Autodesk Inventor part; units mm, degrees
ref_plane "YZ Plane" through (0, 0, 0) normal (1, 0, 0) x (0, 1, 0)
ref_plane "XZ Plane" through (0, 0, 0) normal (0, 1, 0) x (-1, 0, 0)
ref_plane "XY Plane" through (0, 0, 0) normal (0, 0, 1) x (1, 0, 0)
sketch "Sketch1" plane through (0, 0, 0) normal (0, 0, 1) x (1, 0, 0)
  line L0 (-7.3323, 0) -> (-3.6662, 6.35)
  line L1 (-3.6662, 6.35) -> (3.6662, 6.35)
  line L2 (3.6662, 6.35) -> (7.3323, 0)
  line L3 (7.3323, 0) -> (3.6662, -6.35)
  line L4 (3.6662, -6.35) -> (-3.6662, -6.35)
  line L5 (-3.6662, -6.35) -> (-7.3323, 0)
  circle A0 centre (0, 6.35) radius 1.524
  circle A1 centre (-5.4993, 3.175) radius 1.524
  circle A2 centre (-5.4993, -3.175) radius 1.524
  circle A3 centre (0, -6.35) radius 1.524
  circle A4 centre (5.4993, -3.175) radius 1.524
  circle A5 centre (5.4993, 3.175) radius 1.524
  circle A6 centre (0, 0) radius 2.9337
  point P0 (6.2613, 1.8552)
  point P1 (4.7373, 4.4948)
  point P2 (1.524, 6.35)
  point P3 (-1.524, 6.35)
  point P4 (-4.7373, 4.4948)
  point P5 (-6.2613, 1.8552)
  point P6 (-6.2613, -1.8552)
  point P7 (-4.7373, -4.4948)
  point P8 (-1.524, -6.35)
  point P9 (1.524, -6.35)
  point P10 (4.7373, -4.4948)
  point P11 (6.2613, -1.8552)
  dimension "d0" = 12.7
  dimension "d1" = 3.048
  dimension "d4" = 360
  dimension "d6" = 5.8674
extrude "Extrusion1" add sketch "Sketch1" along normal mid plane 60.325 contours L0 A1 L1 A0 L2 A5 L3 A4 L4 A3 L5 A2
properties part number "Configurable Kitbot Churro" material "Aluminum"
For this review, take the finished solid that the model builds, in its own axes (mm). Give positions to 0.01 mm unless a question says otherwise; leave off trailing zeros. Loops run counter-clockwise (first coordinate to the right, second up) from the corner with the lowest first, then second, coordinate; pieces in that order, holes last. Notation, with made-up numbers: M 78,-2.5 L 109,-2.5 A28 ccw 109,30.5 Z; hole C 17,-30.75 d4. An arc over 180 degrees is marked long. Put each result on its own line as item: value. Start each with the question number.
(1) Add section D-D, the plane y = 3.5. Write out the cut boundary in (x, z), then the cut area to 3 significant figures.
(2) Add section A-A, the plane z = 11. Write out the cut boundary in (x, y) (3 decimals).
(3) Wall thickness on L1, parallel to Y at x = 0, z = -17; L2, parallel to Y at x = -2.5, z = -21; L3, parallel to X at y = 5.75, z = 21.5: over which ranges is each line inside the solid? List them lowest first.
(4) For pin 1 (2 mm diameter, centred on y = -4.5, z = 4.5, fed in from -X); pin 2 (1.5 mm diameter, centred on y = 3.5, z = 22, fed in from +X), all flat-tipped, find the tip position at first contact; note any pin that passes through.
(5) Add section B-B, the plane x = 0. Write out the cut boundary in (y, z), then the cut area to 3 significant figures.
(6) Add section C-C, the plane x = -2.25. Write out the cut boundary in (y, z), then the cut area to 3 significant figures.
(7) The part is to be moulded in two halves that separate along Y. For faces 1 (the flat face through (3.2, 0.1, -30.162)), 2 (the flat face through (4.21, -5.41, -0.42)), 3 (the cylindrical face through (4.2, 2.38, -0.42)), 4 (the cylindrical face through (-4.163, 2.442, -0.422)), say which applies: +Y half, -Y half, draft (parallel to the pull), parting line (faces both ways), or undercut.
Result:
1. outline: M -4.01,-30.16 L 4.01,-30.16 L 4.01,30.16 L -4.01,30.16 Z
1. area: 484 mm^2
2. outline: M -7.332,0 L -6.261,-1.855 A1.524 cw -4.737,-4.495 L -3.666,-6.35 L -1.524,-6.35 A1.524 cw 1.524,-6.35 L 3.666,-6.35 L 4.737,-4.495 A1.524 cw 6.261,-1.855 L 7.332,0 L 6.261,1.855 A1.524 cw 4.737,4.495 L 3.666,6.35 L 1.524,6.35 A1.524 cw -1.524,6.35 L -3.666,6.35 L -4.737,4.495 A1.524 cw -6.261,1.855 Z; hole C 0,0 d5.867
3. L1: y = -4.83 to -2.93, 2.93 to 4.83
3. L2: y = -6.35 to -1.54, 1.54 to 6.35
3. L3: x = -4.01 to -1.4, 1.4 to 4.01
4. pin 1: stops at x = -4.74
4. pin 2: stops at x = 4.42
5. outline: M -4.83,-30.16 L -2.93,-30.16 L -2.93,30.16 L -4.83,30.16 Z; M 2.93,-30.16 L 4.83,-30.16 L 4.83,30.16 L 2.93,30.16 Z
5. area: 228 mm^2
6. outline: M -6.35,-30.16 L -1.88,-30.16 L -1.88,30.16 L -6.35,30.16 Z; M 1.88,-30.16 L 6.35,-30.16 L 6.35,30.16 L 1.88,30.16 Z
6. area: 539 mm^2
7. face 1: draft
7. face 2: -Y half
7. face 3: undercut
7. face 4: undercut
